```python
from build123d import *

# Parameters (mm, degrees)
F0_W          = 152.4
F0_H          = 111.3182650085
F1_DEPTH      = 25.4
F1_DEPTH_BACK = 25.4
F2_R          = 38.1
F3_DEPTH      = 50.801
F4_R          = 12.7
F4_R_2        = 5.4393571469
F5_DEPTH      = 25.4


with BuildPart() as f1:
    # F0 (on Front) → F1 (new body, two sides)
    with BuildSketch(Plane.XZ) as f1_sk:
        with Locations((5.7149976492, -6.166184321)):
            Rectangle(F0_W, F0_H)
    extrude(amount=F1_DEPTH)
    extrude(f1_sk.sketch, amount=-F1_DEPTH_BACK)

    # F2 (on face) → F3 (cut, through all)
    with BuildSketch(Plane.XZ.offset(25.4)):
        Circle(F2_R)
    extrude(amount=-F3_DEPTH, mode=Mode.SUBTRACT)

    # F4 (on face) → F5 (cut)
    with BuildSketch(Plane.XY.offset(49.4929481832)):
        with Locations((-1.347124782, 13.6859212071)):
            Circle(F4_R)
        with Locations((22.58563655, 11.8023242822)):
            Circle(F4_R_2)
    extrude(amount=-F5_DEPTH, mode=Mode.SUBTRACT)


solid = f1.part
```
Can you work these out from the model? Positions are in its coordinate system, mm. Round coordinates to 2 decimals unless told otherwise and drop trailing zeros. Loops run counter-clockwise (first coordinate to the right, second up) from the corner with the lowest first, then second, coordinate; pieces in that order, holes last. Notation, with made-up numbers: M 69,-28 L 127,-28 A10 ccw 127,-24 Z; hole C 76.5,-39 d3. An arc over 180 degrees is marked long. Answer in a Markdown table with one row per item.
1. If we section it at A-A, the plane z = 0: Please give me the cut outline in (x, y) (3 decimals), plus the area to 3 significant figures.
Established:
| item | result |
|---|---|
| outline | M -70.485,-25.4 L -38.1,-25.4 L -38.1,25.4 L -70.485,25.4 Z; M 38.1,-25.4 L 81.915,-25.4 L 81.915,25.4 L 38.1,25.4 Z |
| area | 3,870 mm² |
2. If we section it at D-D, the plane z = 42: Please give me the cut outline in (x, y) (3 decimals).
Established:
| item | result |
|---|---|
| outline | M -70.485,-25.4 L 81.915,-25.4 L 81.915,25.4 L 3.559,25.4 A12.7 cw long -6.253,25.4 L -70.485,25.4 Z; hole C 22.586,11.802 d10.879 |
3. Thinking about a two-plate mould opening in Y: for faces 1 (the face through (-1.835, 0.995, 42.552)), 2 (the face through (39, -25.4, -5)), 3 (the face through (27.61, 9.72, 40.45)), 4 (the face through (81.915, 0, -7)), which applies, pulls with the +Y half, pulls with the -Y half, needs draft (parallel to the pull), parting line crosses it, or undercut?
Established:
| item | result |
|---|---|
| face 1 | undercut |
| face 2 | pulls with the -Y half |
| face 3 | undercut |
| face 4 | needs draft |
4. Please list where these lines run through material, in increasing order: line 1 (X direction, y = 3.5, z = 1.5) (3 decimals); line 2 (Z direction, x = 0, y = -12); line 3 (X direction, y = -5, z = -33.5) (3 decimals). Write a range as from..to.
Established:
| item | result |
|---|---|
| line 1 | -70.485..-38.07, 38.07..81.915 |
| line 2 | -61.83..-38.1, 38.1..49.49 |
| line 3 | -70.485..-18.148, 18.148..81.915 |
5. If we section it at B-B, the plane y = -9: Please give me the cut outline in (x, z) (3 decimals), plus the area to 3 significant figures.
Established:
| item | result |
|---|---|
| outline | M -70.485,-61.825 L 81.915,-61.825 L 81.915,49.493 L -70.485,49.493 Z; hole C 0,0 d76.2 |
| area | 12,400 mm² |
6. If we section it at C-C, the plane x = 0: Please give me the cut outline in (y, z), plus the area to 3 significant figures.
Established:
| item | result |
|---|---|
| outline | M -25.4,-61.83 L 25.4,-61.83 L 25.4,-38.1 L -25.4,-38.1 Z; M -25.4,38.1 L 1.06,38.1 L 1.06,49.49 L -25.4,49.49 Z |
| area | 1,510 mm² |
